Can you work these out from the model? Positions are in its coordinate system, mm. A direction names the side the tool comes from. Give positions to 0.01 mm unless a question says otherwise; leave off trailing zeros. Loops run counter-clockwise (first coordinate to the right, second up) from the corner with the lowest first, then second, coordinate; pieces in that order, holes last. Notation, with made-up numbers: (-21.75, 50) -> (31.25, 50) arc R16 cw to (31.25, 58) -> close; hole circle Ø1 at (-29, -12.5). An arc over 180 degrees is marked (long way). Return JSON: item names as keys, results as strings. Group by question number.
Q1. Thinking about a two-plate mould opening in X: for faces 1 (the flat face through (0, 49, -39)), 2 (the flat face through (-148, 95.25, -46)), 3 (the cylindrical face through (-288.88, 34.24, -33.06)), which applies, pulls with the +X half, pulls with the -X half, needs draft (parallel to the pull), parting line crosses it, or undercut?
Q2. Suppose I cut it at C-C, the plane z = -38.1. Please give me the cut outline in (x, y) (3 decimals), and give its area (3 significant figures).
Q3. Suppose I cut it at B-B, the plane x = -146.05. Please give me the cut outline in (y, z), and give its area (3 significant figures).
Q4. Suppose I cut it at D-D, the plane y = 16.5. Please give me the cut outline in (x, z).
Q5. Which directions (+Z, -Z, +X, -X, +Y, -Y) give clear straight access to the entire face, cutting with the end or side of a thin tool? Please do faces 4 (the cylindrical face through (-3.13, 7.24, -68.56)), 5 (the flat face through (-285.75, 45, -38)).
Q6. Suppose I cut it at A-A, the plane y = 38.1. Please give me the cut outline in (x, z), and give its area (3 significant figures).
Q7. I need wall thicknesses on line 1 along X through (y, z) = (70, -67.5); line 2 along X through (y, z) = (99, -38); line 3 along Y through (x, z) = (-287.5, -38.1). Which ranges of each line are inside material? Lowest first, please. Write a range as [from, to].
Q8. Will these pins go through, and if not, where does the flat tip stop? pin 1 (5 mm diameter, centred on x = -44.5, y = 90.5, fed in from -Z); pin 2 (1 mm diameter, centred on x = -35, z = -59, fed in from -Y).
Autodesk Inventor part; units mm, degrees
ref_plane "YZ Plane" through (0, 0, 0) normal (1, 0, 0) x (0, 1, 0)
ref_plane "XZ Plane" through (0, 0, 0) normal (0, 1, 0) x (-1, 0, 0)
ref_plane "XY Plane" through (0, 0, 0) normal (0, 0, 1) x (1, 0, 0)
sketch "Sketch1" plane through (0, 0, 0) normal (0, 1, 0) x (-1, 0, 0)
  line L0 (0, 0) -> (292.1, 0)
  line L1 (292.1, 0) -> (292.1, -76.2)
  line L2 (292.1, -76.2) -> (0, -76.2)
  line L3 (0, -76.2) -> (0, 0)
  circle A0 centre (146.05, -38.1) radius 6.35
  point P0 (292.1, -38.1)
  dimension "d0" = 292.1
  dimension "d1" = 76.2
  dimension "d27" = 12.7
  dimension "d28" = 38.1
  dimension "d45" = 146.05
  dimension "d46" = 146.05
extrude "Extrusion4" add sketch "Sketch1" along normal blind 101.6
sketch "Sketch4" plane through (-292.1, 0, 0) normal (0, 0, 1) x (1, 0, 0)
  line L0 (285.75, -50.8) -> (6.35, -50.8)
  line L1 (6.35, -50.8) -> (6.35, 95.25)
  line L2 (6.35, 95.25) -> (285.75, 95.25)
  line L3 (285.75, 95.25) -> (285.75, -50.8)
  line L4 (0, 101.6) -> (292.1, 101.6)
  line L5 (292.1, 0) -> (292.1, 101.6)
  line L6 (0, 0) -> (0, 101.6)
  point P0 (0, 50.8)
  dimension "d32" = 6.35
  dimension "d33" = 6.35
  dimension "d34" = 6.35
  dimension "d43" = 146.05
extrude "Extrusion5" cut sketch "Sketch4" against normal blind 119.0625
fillet "Fillet4" radius 25.4 4 edges at (-288.925, 0, 0) (-288.925, 0, -76.2) (-3.175, 0, 0) (-3.175, 0, -76.2)
sketch "Sketch5" plane through (0, 101.6, 0) normal (1, 0, 0) x (0, 0, -1)
  circle A0 centre (38.1, -63.5) radius 6.35
  line L0 (0, 0) -> (76.2, 0)
  line L1 (0, -76.2) -> (0, 0)
  point P0 (0, -101.6)
  dimension "d38" = 12.7
  dimension "d39" = 63.5
  dimension "d40" = 38.1
extrude "Extrusion6" cut sketch "Sketch5" against normal blind 330.2
fillet "Fillet5" radius 3.175 4 edges at (-292.1, 101.6, -38.1) (-285.75, 95.25, -38.1) (0, 101.6, -38.1) (-6.35, 95.25, -38.1)
properties part number "Bracket" material "Aluminum 6061"
Ans:
{
 "1": {"face 1": "pulls with the +X half", "face 2": "undercut", "face 3": "needs draft"},
 "2": {"outline": "(-292.1, 0) -> (-285.75, 0) -> (-285.75, 31.75) -> (-292.1, 31.75) -> close; (-292.1, 44.45) -> (-285.75, 44.45) -> (-285.75, 92.075) arc R3.175 cw to (-282.575, 95.25) -> (-152.4, 95.25) -> (-152.4, 101.6) -> (-288.925, 101.6) arc R3.175 ccw to (-292.1, 98.425) -> close; (-139.7, 95.25) -> (-9.525, 95.25) arc R3.175 cw to (-6.35, 92.075) -> (-6.35, 44.45) -> (0, 44.45) -> (0, 98.425) arc R3.175 ccw to (-3.175, 101.6) -> (-139.7, 101.6) -> close; (-6.35, 0) -> (0, 0) -> (0, 31.75) -> (-6.35, 31.75) -> close", "area": "2,820 mm^2"},
 "3": {"outline": "(95.25, -76.2) -> (101.6, -76.2) -> (101.6, -44.45) -> (95.25, -44.45) -> close; (95.25, -31.75) -> (101.6, -31.75) -> (101.6, 0) -> (95.25, 0) -> close", "area": "403 mm^2"},
 "4": {"outline": "(-292.1, -74.59) -> (-285.75, -74.59) -> (-285.75, -1.61) -> (-292.1, -1.61) -> close; (-6.35, -74.59) -> (0, -74.59) -> (0, -1.61) -> (-6.35, -1.61) -> close"},
 "5": {"face 4": "-Z, +X, -X, -Y", "face 5": "+Z, -Z, -Y"},
 "6": {"outline": "(-292.1, -76.2) -> (-285.75, -76.2) -> (-285.75, -44.45) -> (-292.1, -44.45) -> close; (-292.1, -31.75) -> (-285.75, -31.75) -> (-285.75, 0) -> (-292.1, 0) -> close; (-6.35, -76.2) -> (0, -76.2) -> (0, -44.45) -> (-6.35, -44.45) -> close; (-6.35, -31.75) -> (0, -31.75) -> (0, 0) -> (-6.35, 0) -> close", "area": "806 mm^2"},
 "7": {"line 1": "x = [-292.1, -285.75], [-6.35, 0]", "line 2": "x = [-292.05, -152.4], [-139.7, -0.05]", "line 3": "y = [0, 31.75], [44.45, 101.6]"},
 "8": {"pin 1": "passes through", "pin 2": "stops at y = 95.25"}
}
